from build123d import *

# Parameters (mm, degrees)
SKETCH1_W           = 52
SKETCH1_H           = 65
SKETCH1_W_2         = 19
SKETCH1_H_2         = 25
BOSS_EXTRUDE1_DEPTH = 3
CUT_EXTRUDE1_DEPTH  = 2.15
HOLE1_D             = 3.2
FILLET1_R           = 10


with BuildPart() as part:
    # Sketch1 → Boss-Extrude1 (new body)
    with BuildSketch(Plane(origin=(0, 0, 0), x_dir=(1, 0, 0), z_dir=(0, 1, 0))):
        with Locations((-26, -32.5)):
            Rectangle(SKETCH1_W, SKETCH1_H)
        with Locations((-61.5, -32.5)):
            Rectangle(SKETCH1_W_2, SKETCH1_H_2)
    extrude(amount=BOSS_EXTRUDE1_DEPTH)

    # Sketch2 → Cut-Extrude1 (cut)
    with BuildSketch(Plane.XZ):
        Polygon((-3.975, 48.253515436), (-3.975, 51.746484564), (-7, 53.492969129), (-10.025, 51.746484564), (-10.025, 48.253515436), (-7, 46.507030871), align=None)
        Polygon((-33.507030871, 60), (-35.253515436, 63.025), (-38.746484564, 63.025), (-40.492969129, 60), (-38.746484564, 56.975), (-35.253515436, 56.975), align=None)
        Polygon((-18.746484564, 56.975), (-15.253515436, 56.975), (-13.507030871, 60), (-15.253515436, 63.025), (-18.746484564, 63.025), (-20.492969129, 60), align=None)
        Polygon((-15.253515436, 46.975), (-13.507030871, 50), (-15.253515436, 53.025), (-18.746484564, 53.025), (-20.492969129, 50), (-18.746484564, 46.975), align=None)
        Polygon((-35.253515436, 46.975), (-33.507030871, 50), (-35.253515436, 53.025), (-38.746484564, 53.025), (-40.492969129, 50), (-38.746484564, 46.975), align=None)
        Polygon((-35.253515436, 11.975), (-33.507030871, 15), (-35.253515436, 18.025), (-38.746484564, 18.025), (-40.492969129, 15), (-38.746484564, 11.975), align=None)
        Polygon((-15.253515436, 11.975), (-13.507030871, 15), (-15.253515436, 18.025), (-18.746484564, 18.025), (-20.492969129, 15), (-18.746484564, 11.975), align=None)
        Polygon((-13.507030871, 5), (-15.253515436, 8.025), (-18.746484564, 8.025), (-20.492969129, 5), (-18.746484564, 1.975), (-15.253515436, 1.975), align=None)
        Polygon((-38.746484564, 8.025), (-40.492969129, 5), (-38.746484564, 1.975), (-35.253515436, 1.975), (-33.507030871, 5), (-35.253515436, 8.025), align=None)
        Polygon((-23.975, 48.253515436), (-23.975, 51.746484564), (-27, 53.492969129), (-30.025, 51.746484564), (-30.025, 48.253515436), (-27, 46.507030871), align=None)
        Polygon((-23.975, 16.746484564), (-27, 18.492969129), (-30.025, 16.746484564), (-30.025, 13.253515436), (-27, 11.507030871), (-23.975, 13.253515436), align=None)
        Polygon((-58.975, 34.246484564), (-62, 35.992969129), (-65.025, 34.246484564), (-65.025, 30.753515436), (-62, 29.007030871), (-58.975, 30.753515436), align=None)
        Polygon((-7, 18.492969129), (-10.025, 16.746484564), (-10.025, 13.253515436), (-7, 11.507030871), (-3.975, 13.253515436), (-3.975, 16.746484564), align=None)
    extrude(amount=-CUT_EXTRUDE1_DEPTH, mode=Mode.SUBTRACT)

    # Hole1 (through all)
    with Locations(Plane(origin=(-37, 0, 5), x_dir=(0, 0, -1), z_dir=(0, -1, 0))):
        with Locations((0, 0), (-10, 0), (-10, 20), (0, 20), (-10, 10), (-45, 10), (-45, 20), (-55, 20), (-55, 0), (-45, 0), (-27.5, -25), (-10, 30), (-45, 30)):
            Hole(HOLE1_D / 2)

    # Fillet1
    fillet1_edges = [part.edges().sort_by_distance(p)[0] for p in [
        (-71, 1.5, 45),
        (-71, 1.5, 20),
    ]]
    fillet(fillet1_edges, radius=FILLET1_R)


solid = part.part
Geometry check sheet. Reference: the model listing, model coordinates, mm. A direction names the side the tool comes from. Coordinates: 2 decimals unless noted, no trailing zeros. Order: outer loops, then holes, each group sorted by start corner. A loop starts at its lowest first (then second) coordinate and runs counter-clockwise, first axis right, second up. Notation, with made-up numbers: (-20.5, -29) - (16.5, -29) arc R26 ccw to (16.5, 3) - close; hole circle Ø8 at (64.25, 72). An arc over 180 degrees is marked (long way). One line per item, written item: value.
(1) Sectioned sample at B-B (x = -56). Enter the section's corners in (y, z), and give its area (3 significant figures).
Data:
outline: (0, 20) - (3, 20) - (3, 45) - (0, 45) - close
area: 75.0 mm^2
(2) Access from +Z, -Z, +X, -X, +Y, -Y to the whole of each face (thin tool, end or side, straight path). Record for faces 1 (the face through (-38.42, 2.58, 5.74)), 2 (the face through (-28.53, 1.06, 47.39)).
Data:
face 1: +Y, -Y
face 2: -Y
(3) Sectioned sample at A-A (y = 1.25). Count the separate pieces of the cut face and the enclosed holes in it, and give its area (3 significant figures).
Data:
separate pieces: 1
enclosed holes: 13
area: 3,400 mm^2
(4) Release check for a two-part mould opening along X. For faces 3 (the face through (-26, 1, 0)), 4 (the face through (-19.61, 1.06, 61.53)) record: +X half, -X half, draft (parallel to the pull), parting line (faces both ways), or undercut.
Data:
face 3: draft
face 4: undercut
(5) Depth check by flat-ended pin: pin 1 Ø0.6 at (y, z) = (0.5, 50.5) entering from -X; pin 2 Ø2.5 at (x, z) = (-37, 15) entering from -Y; pin 3 Ø1.5 at (x, y) = (-57, 1) entering from +Z. Enter the tip coordinate at first touch or a pass-through.
Data:
pin 1: stops at x = -52
pin 2: passes through
pin 3: stops at z = 45
(6) Thickness scan on probe 1 along X at (y, z) = (2.45, 50); probe 2 along Z at (x, y) = (-18.5, 0.4) (3 decimals); probe 3 along X at (y, z) = (2.7, 5). Record the ranges inside material, lowest first. Write a range as from..to.
Data:
probe 1: x = -52..-38.6, -35.4..-28.6, -25.4..-18.6, -15.4..-8.6, -5.4..0
probe 2: z = 0..1.975, 8.025..11.975, 18.025..46.975, 53.025..56.975, 63.025..65
probe 3: x = -52..-38.6, -35.4..-18.6, -15.4..0
